Work out the finished part from the listing and answer in its coordinate system (mm). Face numbers are marked on the shaded views. A direction names the side the tool comes from. Give positions to 0.01 mm unless a question says otherwise; leave off trailing zeros. Loops run counter-clockwise (first coordinate to the right, second up) from the corner with the lowest first, then second, coordinate; pieces in that order, holes last. Notation, with made-up numbers: M 87.5,71.5 L 104.5,71.5 A17 cw 104.5,83.5 Z; hole C -37.75,-25.5 d3. An arc over 180 degrees is marked long. Answer in a Markdown table with one row per item. Add a question column.
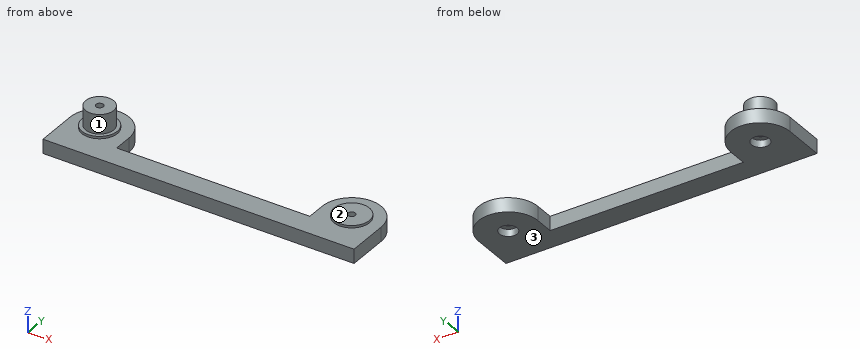
from build123d import *

# Parameters (mm, degrees)
F2_DEPTH  = 6
F3_R      = 7.5
F4_DEPTH  = 1
F5_R      = 5.95
F6_DEPTH  = 8.2
F7_R      = 1.55
F8_DEPTH  = 15.201
F9_R      = 3.75
F10_DEPTH = 3


with BuildPart() as f2:
    # F1 (on Top) → F2 (new body)
    with BuildSketch(Plane.XY):
        with BuildLine():
            Line((-40.941557, -103), (-40.941557, -95))
            ThreePointArc((-40.941557, -95), (-53.441557, -82.5), (-65.941557, -95))
            Line((-65.941557, -95), (-65.941557, -112.5))
            Line((-65.941557, -112.5), (0, -112.5))
            Line((0, -112.5), (65.941557, -112.5))
            Line((65.941557, -112.5), (65.941557, -95))
            ThreePointArc((65.941557, -95), (53.441557, -82.5), (40.941557, -95))
            Line((40.941557, -95), (40.941557, -103))
            Line((40.941557, -103), (0, -103))
            Line((0, -103), (-40.941557, -103))
        make_face()
    extrude(amount=F2_DEPTH)

    # F3 (on face) → F4 (join)
    with BuildSketch(Plane.XY.offset(6)):
        with Locations((-53.441557, -95)):
            Circle(F3_R)
        with Locations((53.441557, -95)):
            Circle(F3_R)
    extrude(amount=F4_DEPTH)

    # F5 (on face) → F6 (join)
    with BuildSketch(Plane.XY.offset(7)):
        with Locations((-53.441557, -95)):
            Circle(F5_R)
    extrude(amount=F6_DEPTH)

    # F7 (on face) → F8 (cut, through all)
    with BuildSketch(Plane.XY):
        with Locations((-53.441557, -95)):
            Circle(F7_R)
        with Locations((53.441557, -95)):
            Circle(F7_R)
    extrude(amount=F8_DEPTH, mode=Mode.SUBTRACT)

    # F9 (on face) → F10 (cut)
    with BuildSketch(Plane.XY):
        with Locations((-53.441557, -95)):
            Circle(F9_R)
        with Locations((53.441557, -95)):
            Circle(F9_R)
    extrude(amount=F10_DEPTH, mode=Mode.SUBTRACT)


solid = f2.part
(1) Section B-B, the plane x = -33 is taken. Determine the outline of the cut face in (y, z), and give its area (3 significant figures).
(2) Each of these flat-tipped pins is pushed along its axis until it touches: P1, Ø4.5, axis at x = 54, y = -95.5, coming from the +Z side; P2, Ø1.8, axis at x = 8, z = 2.5, coming from the +Y side; P3, Ø2, axis at x = 53, y = -95.5, coming from the -Z side. Where does it stop, or does it pass through?
(3) Consider line 1 along X through (y, z) = (-95, 4.8); line 2 along Y through (x, z) = (-39, 0.75); line 3 along Z through (x, y) = (43, -96.25). Determine where each line is inside the solid, lowest interval first. Write a range as from..to.
(4) Which of the six approach directions +Z, -Z, +X, -X, +Y, -Y give full straight-line access (tool end or side, diameter ignored) to the marked faces 1, 2 and 3?
(5) Section A-A, the plane z = 10.75 is taken. Determine the outline of the cut face in (x, y), and give its area (3 significant figures).
(6) Section C-C, the plane y = -108.75 is taken. Determine the outline of the cut face in (x, z).
Numbers:
| question | item | result |
|---|---|---|
| 1 | outline | M -112.5,0 L -103,0 L -103,6 L -112.5,6 Z |
| 1 | area | 57.0 mm² |
| 2 | P1 | stops at z = 7 |
| 2 | P2 | stops at y = -103 |
| 2 | P3 | stops at z = 3 |
| 3 | line 1 | x = -65.94..-54.99, -51.89..-40.94, 40.94..51.89, 54.99..65.94 |
| 3 | line 2 | y = -112.5..-103 |
| 3 | line 3 | z = 0..6 |
| 4 | face 1 | +Z |
| 4 | face 2 | +Z, +X, +Y, -Y |
| 4 | face 3 | -Z, +X, -X, +Y, -Y |
| 5 | outline | C -53.44,-95 d11.9; hole C -53.44,-95 d3.1 |
| 5 | area | 104 mm² |
| 6 | outline | M -65.94,0 L 65.94,0 L 65.94,6 L -65.94,6 Z |
